The listing builds one solid part. Answer for the finished solid, in the listing's coordinates (mm). Round coordinates to 2 decimals unless told otherwise and drop trailing zeros. Write each loop counter-clockwise with the first axis right and the second up, starting at its lowest first coordinate (ties: lowest second). Pieces come first, ordered by that corner, then holes.
Item 1: Find section C-C on x = -40.75. Give the vertices of the cut face in (y, z), then the cut area to 3 significant figures.
Item 2: Find section B-B on y = 9.5. Give the vertices of the cut face in (x, z).
Item 3: Find the intervals of material crossed by probe 1 along X at (y, z) = (9.25, 0.1); probe 2 along Y at (x, z) = (-38, 0.35); probe 3 along X at (y, z) = (7, 0.1), in increasing order.
Item 4: Find section D-D on y = 7.5. Give the vertices of the cut face in (x, z), then the cut area to 3 significant figures.
Item 5: Find section A-A on z = 0.3. Give the vertices of the cut face in (x, y).
```python
from build123d import *

# Parameters (mm, degrees)
PAD002_DEPTH    = 0.4
SKETCH010_W     = 1.6
SKETCH010_H     = 1
POCKET006_DEPTH = 0.401


with BuildPart() as contact:
    # Sketch009 (on Face1 of ShapeBinder) → Pad002 (new body)
    with BuildSketch(Plane(origin=(0, 0, 0), x_dir=(1, 0, 0), z_dir=(0, 0, -1))):
        Polygon((36.05, 11.4), (38.55, 11.4), (38.55, 12.8), (42.95, 12.8), (42.95, 6.3), (38.55, 6.3), (38.55, 7.7), (36.05, 7.7), align=None)
    extrude(amount=-PAD002_DEPTH)

    # Sketch010 (on Face9 of Pad002) → Pocket006 (cut, through all)
    with BuildSketch(Plane(origin=(0, 0, 0), x_dir=(1, 0, 0), z_dir=(0, 0, -1))):
        with Locations((40.55, 9.55)):
            Rectangle(SKETCH010_W, SKETCH010_H)
    extrude(amount=-POCKET006_DEPTH, mode=Mode.SUBTRACT)


with BuildPart() as contact_mirrored:
    # mirror: instance of contact
    add(contact.part.mirror(Plane(origin=(0, 19.85, 7), x_dir=(0, 1, 0), z_dir=(-1, 0, 0))))


with BuildPart() as contact_mirrored_mirrored:
    # mirror001: instance of contact (mirrored)
    add(contact_mirrored.part.mirror(Plane(origin=(-38.55, 0, 15), x_dir=(-1, 0, 0), z_dir=(0, -1, 0))))


solid = contact_mirrored_mirrored.part
```
Check values:
1. outline: (6.3, 0) - (9.05, 0) - (9.05, 0.4) - (6.3, 0.4) - close; (10.05, 0) - (12.8, 0) - (12.8, 0.4) - (10.05, 0.4) - close
1. area: 2.20 mm2
2. outline: (-42.95, 0) - (-41.35, 0) - (-41.35, 0.4) - (-42.95, 0.4) - close; (-39.75, 0) - (-36.05, 0) - (-36.05, 0.4) - (-39.75, 0.4) - close
3. probe 1: x = -42.95 to -41.35, -39.75 to -36.05
3. probe 2: y = 7.7 to 11.4
3. probe 3: x = -42.95 to -38.55
4. outline: (-42.95, 0) - (-38.55, 0) - (-38.55, 0.4) - (-42.95, 0.4) - close
4. area: 1.76 mm2
5. outline: (-42.95, 6.3) - (-38.55, 6.3) - (-38.55, 7.7) - (-36.05, 7.7) - (-36.05, 11.4) - (-38.55, 11.4) - (-38.55, 12.8) - (-42.95, 12.8) - close; hole (-41.35, 9.05) - (-39.75, 9.05) - (-39.75, 10.05) - (-41.35, 10.05) - close
